CAD build for the part. Positions are in the model's coordinates, mm. A direction names the side the tool comes from. Round coordinates to 2 decimals unless told otherwise and drop trailing zeros. Loops run counter-clockwise (first coordinate to the right, second up) from the corner with the lowest first, then second, coordinate; pieces in that order, holes last. Notation, with made-up numbers: M -24,34 L 22,34 A12 cw 22,52 Z; hole C 9.25,84.5 d3. An arc over 180 degrees is marked long. Use one line per item in the form item = value.
from build123d import *

# Parameters (mm, degrees)
SKIZZE1_W                       = 20
SKIZZE1_H                       = 38.3
SKIZZE1_R                       = 1.65
SKIZZE1_W_2                     = 12.5
SKIZZE1_H_2                     = 0.8
AUFSATZ_LINEAR_AUSTRAGEN1_DEPTH = 12
SCHNITT_LINEAR_AUSTRAGEN2_DEPTH = 45.842948164


with BuildPart() as part:
    # Skizze1 → Aufsatz-Linear austragen1 (new body)
    with BuildSketch(Plane(origin=(0, 0, 0), x_dir=(0, 0, -1), z_dir=(1, 0, 0))):
        with Locations((10, 19.15)):
            Rectangle(SKIZZE1_W, SKIZZE1_H)
        with Locations((5, 33.8)):
            Circle(SKIZZE1_R, mode=Mode.SUBTRACT)
        with Locations((15, 33.8)):
            Circle(SKIZZE1_R, mode=Mode.SUBTRACT)
        with Locations((10, 3.4)):
            Rectangle(SKIZZE1_W_2, SKIZZE1_H_2, mode=Mode.SUBTRACT)
        with Locations((10, 7.2)):
            Rectangle(SKIZZE1_W_2, SKIZZE1_H_2, mode=Mode.SUBTRACT)
        with Locations((10, 11)):
            Rectangle(SKIZZE1_W_2, SKIZZE1_H_2, mode=Mode.SUBTRACT)
    extrude(amount=AUFSATZ_LINEAR_AUSTRAGEN1_DEPTH)

    # Skizze2 → Schnitt-Linear austragen2 (cut, through all)
    with BuildSketch(Plane.XY):
        with BuildLine():
            Line((3.5, 38.3), (8.5, 38.3))
            Line((8.5, 38.3), (8.5, 27.458312395))
            ThreePointArc((8.5, 27.458312395), (6, 22.8), (3.5, 27.458312395))
            Line((3.5, 27.458312395), (3.5, 38.3))
        make_face()
    extrude(amount=-SCHNITT_LINEAR_AUSTRAGEN2_DEPTH, mode=Mode.SUBTRACT)


solid = part.part
1. Cut at B-B on z = -12.75. Write the cut outline in (x, y).
Completed:
outline = M 0,0 L 12,0 L 12,3 L 0,3 Z; M 0,3.8 L 12,3.8 L 12,6.8 L 0,6.8 Z; M 0,7.6 L 12,7.6 L 12,10.6 L 0,10.6 Z; M 0,11.4 L 12,11.4 L 12,38.3 L 8.5,38.3 L 8.5,27.46 A3 cw long 3.5,27.46 L 3.5,38.3 L 0,38.3 Z
2. Pull direction X, two halves, no side cores. Call faces 1 (the face through (12, 19, -10)), 2 (the face through (6.1, 22.8, -9.9)), 3 (the face through (1.726, 34.915, -3.784)): +X half, -X half, draft (parallel to the pull), parting line (faces both ways), or undercut.
Completed:
face_1 = +X half
face_2 = undercut
face_3 = draft
3. Cut at A-A on y = 36.5. Write the cut outline in (x, z), and give its area (3 significant figures).
Completed:
outline = M 0,-20 L 3.5,-20 L 3.5,0 L 0,0 Z; M 8.5,-20 L 12,-20 L 12,0 L 8.5,0 Z
area = 140 mm2
4. Cut at C-C on z = -5. Write the cut outline in (x, y), and give its area (3 significant figures).
Completed:
outline = M 0,0 L 12,0 L 12,3 L 0,3 Z; M 0,3.8 L 12,3.8 L 12,6.8 L 0,6.8 Z; M 0,7.6 L 12,7.6 L 12,10.6 L 0,10.6 Z; M 0,11.4 L 12,11.4 L 12,32.15 L 8.5,32.15 L 8.5,27.46 A3 cw long 3.5,27.46 L 3.5,32.15 L 0,32.15 Z; M 0,35.45 L 3.5,35.45 L 3.5,38.3 L 0,38.3 Z; M 8.5,35.45 L 12,35.45 L 12,38.3 L 8.5,38.3 Z
area = 330 mm2
5. Cut at D-D on x = 6. Write the cut outline in (y, z), and give its area (3 significant figures).
Completed:
outline = M 0,-20 L 22.8,-20 L 22.8,0 L 0,0 Z; hole M 3,-16.25 L 3.8,-16.25 L 3.8,-3.75 L 3,-3.75 Z; hole M 6.8,-16.25 L 7.6,-16.25 L 7.6,-3.75 L 6.8,-3.75 Z; hole M 10.6,-16.25 L 11.4,-16.25 L 11.4,-3.75 L 10.6,-3.75 Z
area = 426 mm2
6. Tool access for faces 4 (the face through (10, 38.3, -10)), 5 (the face through (6, 11, -16.25)), 6 (the face through (8.5, 33, -10)): list every direction of +Z, -Z, +X, -X, +Y, -Y with a clear straight run to the whole face (end or side of a thin tool).
Completed:
face_4 = +Z, -Z, +X, -X, +Y
face_5 = +X, -X
face_6 = +Z, -Z, +Y
7. Probe line 1 along Y through (x, z) = (9.9, -5); line 2 along Y through (x, z) = (6, -5.75); line 3 along Z through (x, y) = (2.3, 33.8). List the from-to ranges inside material, lowest first. Write a range as from..to.
Completed:
line_1 = 0..3, 3.8..6.8, 7.6..10.6, 11.4..32.15, 35.45..38.3
line_2 = 0..3, 3.8..6.8, 7.6..10.6, 11.4..22.8
line_3 = -20..-16.65, -13.35..-6.65, -3.35..0
8. Drop a flat-ended pin along its axis: P1, Ø3.5, axis at x = 6, y = 25.8, coming from the +Z side. Give the stop position or say it passes through.
Completed:
P1 = through
